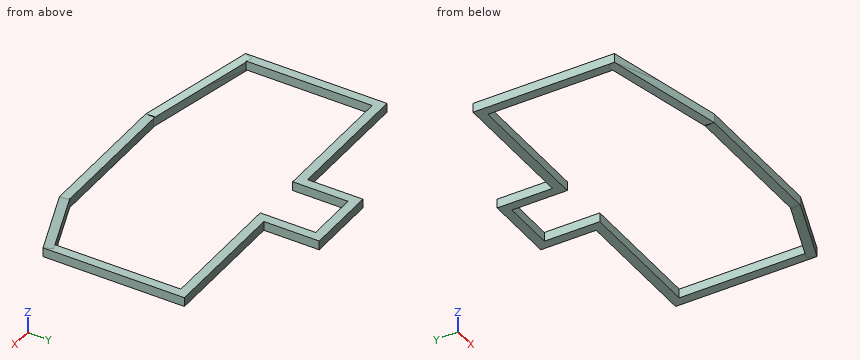
Autodesk Inventor part; units mm, degrees
ref_plane "YZ Plane" through (0, 0, 0) normal (1, 0, 0) x (0, 1, 0)
ref_plane "XZ Plane" through (0, 0, 0) normal (0, 1, 0) x (-1, 0, 0)
ref_plane "XY Plane" through (0, 0, 0) normal (0, 0, 1) x (1, 0, 0)
sketch "Sketch1" plane through (0, 0, 0) normal (0, 0, 1) x (1, 0, 0)
  line L0 (-107.9, 41.925) -> (107.9, -41.925) construction
  line L1 (107.9, 41.925) -> (-107.9, -41.925) construction
  line L2 (-114.4, -47.125) -> (-114.4, 47.125)
  line L3 (114.4, 47.125) -> (114.4, -47.125)
  line L4 (114.4, -47.125) -> (-114.4, 47.125) construction
  line L5 (-114.4, -47.125) -> (114.4, 47.125) construction
  line L6 (-22.1, 47.125) -> (-22.1, 86.125)
  line L7 (-22.1, 86.125) -> (22.1, 86.125)
  line L8 (22.1, 86.125) -> (22.1, 47.125)
  line L9 (22.1, 47.125) -> (114.4, 47.125)
  line L10 (-22.1, 47.125) -> (-114.4, 47.125)
  line L11 (114.4, -47.125) -> (49.4, -75.4283)
  line L12 (-114.4, -47.125) -> (-49.4, -75.4283)
  line L13 (49.4, -75.4283) -> (-49.4, -75.4283)
  point P0 (0, 0)
  point P1 (0, 0)
  point P2 (0, 80.925)
  point P3 (0, 0)
  point P4 (0, 86.125)
  point P5 (0, 0)
  dimension "Comp" = 215.8
  dimension "Lar" = 83.85
  dimension "d10" = 215.8
  dimension "LarMaior" = 94.25
  dimension "CompMaior" = 228.8
  dimension "d20" = 39
  dimension "d21" = 44.2
  dimension "d25" = 65
  dimension "d27" = 65
  dimension "d28" = 98.8
extrude "Extrusion1" add sketch "Sketch1" along normal blind 6.5
shell "Shell1" thickness 6.5 both sides yes removed faces 2 at (-7.3667, -34.5772, 6.5) at (-7.3667, -34.5772, 0)
sketch "Sketch2" plane through (-50.0769, -78.6783, 0) normal (-0.3992292, -0.9168512, 0) x (0.9168512, -0.3992292, 0)
  line L0 (0, 0) -> (0, -14.3)
  line L1 (-113.4763, 0) -> (-73.7013, 0)
  line L2 (0, -14.3) -> (-73.7013, 0)
  line L3 (-73.7013, 0) -> (0, 0)
  point P0 (14.5024, 0)
  dimension "d32" = 14.3
extrude "Extrusion2" add sketch "Sketch2" against normal blind 6.5
sketch "Sketch3" plane through (-50.0769, -78.6783, 6.5) normal (0, -1, 0) x (1, 0, 0)
  line L0 (0, -20.8002) -> (98.8, -20.8002)
  line L1 (100.2059, -6.5) -> (100.2059, -20.8002)
  line L2 (100.2059, -20.8002) -> (98.8, -20.8002)
  line L3 (0, -6.5) -> (0, 0)
  line L4 (0, -6.5) -> (0, -20.8002)
  line L5 (0, -6.5) -> (100.1538, -6.5)
  line L6 (0, -6.5) -> (100.2059, -6.5)
  line L7 (0, 0) -> (100.1538, 0)
  point P0 (50.0769, -6.5)
  dimension "d35" = 98.8
extrude "Extrusion3" add sketch "Sketch3" against normal blind 6.5
sketch "Sketch4" plane through (117.65, -49.2546, 0) normal (0.3992292, -0.9168512, 0) x (0.9168512, 0.3992292, 0)
  line L0 (-165.5274, -14.3002) -> (-73.6535, -14.3002)
  line L1 (0, 0) -> (0, 6.5)
  line L2 (-73.6535, -14.3002) -> (0, 0)
  line L3 (0, 0) -> (-73.6535, 0)
  line L4 (-73.6535, 0) -> (-73.6535, -14.3002)
  point P0 (-88.2037, 0)
extrude "Extrusion4" add sketch "Sketch4" against normal blind 6.5
sketch "Sketch5" plane through (-50.0769, -78.6783, 6.5) normal (0, -1, 0) x (1, 0, 0)
  line L0 (0, -20.8) -> (0, 0)
  line L1 (100.2009, 0) -> (0, 0)
  line L2 (0, 0) -> (0, -14.3951)
  line L3 (0, -14.3951) -> (100.2009, -14.3951)
  line L4 (100.2009, -14.3951) -> (100.2009, 0)
  point P0 (50.0769, -6.5)
extrude "Extrusion5" cut sketch "Sketch5" against normal blind 6.5
sketch "Sketch6" plane through (-117.65, -49.2546, 0) normal (-0.3992292, -0.9168512, 0) x (0.9168512, -0.3992292, 0)
  line L0 (73.7013, -14.3) -> (73.7013, -7.8951)
  line L1 (0, 0) -> (0, 6.5)
  line L2 (73.7013, -7.8951) -> (0, 6.5)
  line L3 (0, 6.5) -> (73.7013, 6.5)
  line L4 (73.7013, 6.5) -> (73.7013, -7.8951)
  point P0 (88.2037, 0)
extrude "Extrusion6" cut sketch "Sketch6" against normal blind 6.5
sketch "Sketch8" plane through (50.129, -78.6556, -14.2985) normal (0.3992292, -0.9168512, 0) x (0.9168512, 0.3992292, 0)
  line L0 (-0.0136, 6.4034) -> (-91.8829, 6.4034)
  line L1 (-0.0054, 20.7985) -> (73.6445, 20.7985)
  line L2 (-0.0136, 6.4034) -> (73.6445, 20.7985)
  line L3 (73.6445, 20.7985) -> (-0.0136, 20.7985)
  line L4 (69.3853, 20.7985) -> (1.2969, 20.7985)
  line L5 (-0.0136, 20.7985) -> (-0.0136, 6.4034)
  line L6 (0, 0) -> (0, 14.2985)
  point P0 (-14.5592, 14.2985)
extrude "Extrusion7" cut sketch "Sketch8" against normal blind 6.5
properties part number "Buste2-2"
Check sheet for the modelled part. Datum: model origin and axes. Units: mm. Give positions to 0.01 mm unless a question says otherwise; leave off trailing zeros. Write each loop counter-clockwise with the first axis right and the second up, starting at its lowest first coordinate (ties: lowest second). Pieces come first, ordered by that corner, then holes.
Item 1: Cross-section at A-A (y = 13). Enter the section's corners in (x, z).
Item 2: Gauge pin test, flat ends, axial feed: pin 1 (3 mm diameter, centred on x = 55, z = -11, fed in from +Y); pin 2 (2 mm diameter, centred on x = 49.5, z = 2.5, fed in from +Y) (3 decimals); pin 3 (7 mm diameter, centred on x = -21.5, y = -74, fed in from +Z); pin 4 (6 mm diameter, centred on y = 28, z = -0.5, fed in from +X). Record the tip position at first contact, or that the pin passes through.
Item 3: Scan lines: L1, parallel to X at y = 1.5, z = 3.5; L2, parallel to Y at x = 55.5, z = 3.75 (3 decimals). Record each from-to range of solid material in increasing order.
Item 4: Cross-section at D-D (y = -52). Enter the section's corners in (x, z) (3 decimals).
Item 5: Cross-section at C-C (x = 78). Enter the section's corners in (y, z) (3 decimals), and give its area (3 significant figures).
Report:
1. outline: (-117.65, 0) - (-111.15, 0) - (-111.15, 6.5) - (-117.65, 6.5) - close; (111.15, 0) - (117.65, 0) - (117.65, 6.5) - (111.15, 6.5) - close
2. pin 1: stops at y = -68.79
2. pin 2: stops at y = 50.375
2. pin 3: stops at z = -7.9
2. pin 4: stops at x = 117.65
3. L1: x = -117.65 to -111.15, 111.15 to 117.65
3. L2: y = 43.875 to 50.375
4. outline: (-111.345, -1.334) - (-95.064, -4.231) - (-95.064, 2.241) - (-111.345, 5.157) - close; (95.064, -4.233) - (111.345, -1.335) - (111.345, 5.156) - (95.064, 2.239) - close
5. outline: (-66.52, -8.396) - (-59.43, -7.847) - (-59.43, -1.398) - (-66.52, -1.952) - close; (43.875, 0) - (50.375, 0) - (50.375, 6.5) - (43.875, 6.5) - close
5. area: 88.0 mm2
